```python
from build123d import *

# Parameters (mm, degrees)
SKETCH1_W           = 31.8
SKETCH1_H           = 15.8
BOSS_EXTRUDE1_DEPTH = 9.6
SKETCH3_W           = 31.8
SKETCH3_H           = 15.8
BOSS_EXTRUDE2_DEPTH = 1
SKETCH4_R           = 2.4
BOSS_EXTRUDE3_DEPTH = 1.8
SKETCH5_R           = 1.3
CUT_EXTRUDE1_DEPTH  = 1.7
SKETCH6_R           = 3.255
SKETCH6_R_2         = 2.4
SKETCH6_R_3         = 3.225
BOSS_EXTRUDE4_DEPTH = 8.6
SKETCH7_W           = 0.8
SKETCH7_H           = 3.759344576
SKETCH7_H_2         = 3.840900034
BOSS_EXTRUDE5_DEPTH = 6.3


with BuildPart() as part:
    # Sketch1 → Boss-Extrude1 (new body)
    with BuildSketch(Plane(origin=(0, 0, 0), x_dir=(1, 0, 0), z_dir=(0, 1, 0))):
        Rectangle(SKETCH1_W, SKETCH1_H)
        Polygon((-12.3, -6.7), (-14.7, -6.7), (-14.7, -4.3), (-14.5, -4.3), (-14.5, -3.7), (-14.7, -3.7), (-14.7, 3.7), (-14.5, 3.7), (-14.5, 4.3), (-14.7, 4.3), (-14.7, 6.7), (-12.3, 6.7), (-12.3, 6.5), (-11.7, 6.5), (-11.7, 6.7), (-4.3, 6.7), (-4.3, 6.5), (-3.7, 6.5), (-3.7, 6.7), (3.7, 6.7), (3.7, 6.5), (4.3, 6.5), (4.3, 6.7), (11.7, 6.7), (11.7, 6.5), (12.3, 6.5), (12.3, 6.7), (14.7, 6.7), (14.7, 4.3), (14.5, 4.3), (14.5, 3.7), (14.7, 3.7), (14.7, -3.7), (14.5, -3.7), (14.5, -4.3), (14.7, -4.3), (14.7, -6.7), (12.3, -6.7), (12.3, -6.5), (11.7, -6.5), (11.7, -6.7), (4.3, -6.7), (4.3, -6.5), (3.7, -6.5), (3.7, -6.7), (-3.7, -6.7), (-3.7, -6.5), (-4.3, -6.5), (-4.3, -6.7), (-11.7, -6.7), (-11.7, -6.5), (-12.3, -6.5), align=None, mode=Mode.SUBTRACT)
    extrude(amount=BOSS_EXTRUDE1_DEPTH)

    # Sketch3 → Boss-Extrude2 (add)
    with BuildSketch(Plane(origin=(0, 9.6, 0), x_dir=(1, 0, 0), z_dir=(0, 1, 0))):
        Rectangle(SKETCH3_W, SKETCH3_H)
    extrude(amount=-BOSS_EXTRUDE2_DEPTH)

    # Sketch4 → Boss-Extrude3 (add)
    with BuildSketch(Plane(origin=(0, 9.6, 0), x_dir=(1, 0, 0), z_dir=(0, 1, 0))):
        with Locations(Location((-12, 4, 0), (0, 0, 270))):
            Circle(SKETCH4_R)
        with Locations(Location((-4, 4, 0), (0, 0, 270))):
            Circle(SKETCH4_R)
        with Locations(Location((4, 4, 0), (0, 0, 270))):
            Circle(SKETCH4_R)
        with Locations(Location((12, 4, 0), (0, 0, 270))):
            Circle(SKETCH4_R)
        with Locations(Location((-12, -4, 0), (0, 0, 270))):
            Circle(SKETCH4_R)
        with Locations(Location((-4, -4, 0), (0, 0, 270))):
            Circle(SKETCH4_R)
        with Locations(Location((4, -4, 0), (0, 0, 270))):
            Circle(SKETCH4_R)
        with Locations(Location((12, -4, 0), (0, 0, 270))):
            Circle(SKETCH4_R)
    extrude(amount=BOSS_EXTRUDE3_DEPTH)

    # Sketch5 → Cut-Extrude1 (cut)
    with BuildSketch(Plane.XZ.offset(-8.6)):
        with Locations(Location((12, -4, 0), (0, 0, 270))):
            Circle(SKETCH5_R)
        with Locations(Location((12, 4, 0), (0, 0, 270))):
            Circle(SKETCH5_R)
        with Locations(Location((4, -4, 0), (0, 0, 270))):
            Circle(SKETCH5_R)
        with Locations(Location((4, 4, 0), (0, 0, 270))):
            Circle(SKETCH5_R)
        with Locations(Location((-4, 4, 0), (0, 0, 270))):
            Circle(SKETCH5_R)
        with Locations(Location((-4, -4, 0), (0, 0, 270))):
            Circle(SKETCH5_R)
        with Locations(Location((-12, -4, 0), (0, 0, 270))):
            Circle(SKETCH5_R)
        with Locations(Location((-12, 4, 0), (0, 0, 270))):
            Circle(SKETCH5_R)
    extrude(amount=-CUT_EXTRUDE1_DEPTH, mode=Mode.SUBTRACT)

    # Sketch6 → Boss-Extrude4 (add)
    # profile 1 of 3: a face of its own
    with BuildSketch(Plane.XZ.offset(-8.6)):
        with Locations(Location((8, 0, 0), (0, 0, 90))):
            Circle(SKETCH6_R)
        with Locations(Location((8, 0, 0), (0, 0, 90))):
            Circle(SKETCH6_R_2, mode=Mode.SUBTRACT)
    # profile 2 of 3: a face of its own
    with BuildSketch(Plane.XZ.offset(-8.6)):
        with Locations(Location((-8, 0, 0), (0, 0, 90))):
            Circle(SKETCH6_R)
        with Locations(Location((-8, 0, 0), (0, 0, 90))):
            Circle(SKETCH6_R_2, mode=Mode.SUBTRACT)
    # profile 3 of 3: a face of its own
    with BuildSketch(Plane.XZ.offset(-8.6)):
        with Locations(Location((0, 0, 0), (0, 0, 90))):
            Circle(SKETCH6_R_3)
        with Locations(Location((0, 0, 0), (0, 0, 90))):
            Circle(SKETCH6_R_2, mode=Mode.SUBTRACT)
    extrude(amount=BOSS_EXTRUDE4_DEPTH)

    # Sketch7 → Boss-Extrude5 (add)
    with BuildSketch(Plane.XZ.offset(-8.6)):
        with Locations((0, -4.820327712)):
            Rectangle(SKETCH7_W, SKETCH7_H)
        with Locations((0, 4.779549983)):
            Rectangle(SKETCH7_W, SKETCH7_H_2)
    extrude(amount=BOSS_EXTRUDE5_DEPTH)


solid = part.part
```
The listing builds one solid part. Answer for the finished solid, in the listing's coordinates (mm). A direction names the side the tool comes from. Give positions to 0.01 mm unless a question says otherwise; leave off trailing zeros. Order: outer loops, then holes, each group sorted by start corner. A loop starts at its lowest first (then second) coordinate and runs counter-clockwise, first axis right, second up.
Item 1: Given pin 1 Ø4 at (x, z) = (8, -6) entering from +Y; pin 2 Ø0.6 at (x, z) = (0, 5) entering from -Y; pin 3 Ø1.4 at (x, z) = (7.5, 1) entering from -Y, each flat-ended and moving along its own axis, determine where each tip first touches the part or whether it passes through.
From the geometry:
pin 1: stops at y = 9.6
pin 2: stops at y = 2.3
pin 3: stops at y = 8.6
Item 2: Which of the six approach directions +Z, -Z, +X, -X, +Y, -Y give full straight-line access (tool end or side, diameter ignored) to faces 4 (the face through (-12, 11.4, -4)), 5 (the face through (14.024, 10.487, 5.29)), 6 (the face through (-2.024, 4.36, 1.29))?
From the geometry:
face 4: +Z, -Z, +X, -X, +Y
face 5: +Y
face 6: -Y
Item 3: The part is cut by section B-B, the plane x = 8. Give the vertices of the cut face in (y, z) (3 decimals).
From the geometry:
outline: (0, -7.9) - (9.6, -7.9) - (9.6, 7.9) - (0, 7.9) - (0, 6.7) - (8.6, 6.7) - (8.6, 3.255) - (0, 3.255) - (0, 2.4) - (8.6, 2.4) - (8.6, -2.4) - (0, -2.4) - (0, -3.255) - (8.6, -3.255) - (8.6, -6.7) - (0, -6.7) - close
Item 4: The part is cut by section D-D, the plane x = 12. Give the vertices of the cut face in (y, z).
From the geometry:
outline: (0, -7.9) - (9.6, -7.9) - (9.6, -6.4) - (11.4, -6.4) - (11.4, -1.6) - (9.6, -1.6) - (9.6, 1.6) - (11.4, 1.6) - (11.4, 6.4) - (9.6, 6.4) - (9.6, 7.9) - (0, 7.9) - (0, 6.5) - (8.6, 6.5) - (8.6, 5.3) - (10.3, 5.3) - (10.3, 2.7) - (8.6, 2.7) - (8.6, -2.7) - (10.3, -2.7) - (10.3, -5.3) - (8.6, -5.3) - (8.6, -6.5) - (0, -6.5) - close
Item 5: The part is cut by section A-A, the plane y = 3.5. Count the separate pieces of the cut face and the enclosed holes in it, and give its area (3 significant figures).
From the geometry:
separate pieces: 3
enclosed holes: 5
area: 160 mm2
Item 6: For a pull along Z with two mould halves and no side action, classify faces 1 (the face through (1, 4, 6.7)), 2 (the face through (-15.9, 5, 0)), 3 (the face through (8, 4, -6.7)) as pulls with the +Z half, pulls with the -Z half, needs draft (parallel to the pull), parting line crosses it, or undercut.
From the geometry:
face 1: undercut
face 2: needs draft
face 3: undercut
Item 7: Find the intervals of material crossed by probe 1 along X at (y, z) = (9.35, -4); probe 2 along Z at (x, y) = (7.5, 1); probe 3 along X at (y, z) = (5.25, -2.75), in increasing order.
From the geometry:
probe 1: x = -15.9 to -13.3, -10.7 to -5.3, -2.7 to 2.7, 5.3 to 10.7, 13.3 to 15.9
probe 2: z = -7.9 to -6.7, -3.22 to -2.35, 2.35 to 3.22, 6.7 to 7.9
probe 3: x = -15.9 to -14.7, -9.74 to -6.26, -1.68 to 1.68, 6.26 to 9.74, 14.7 to 15.9
